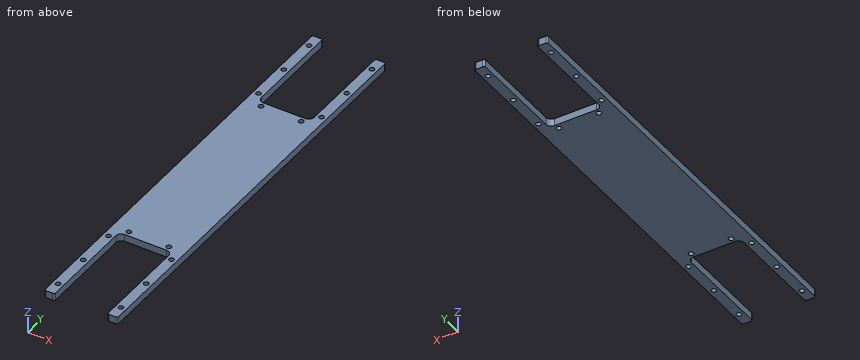
Autodesk Inventor part; units mm, degrees
ref_plane "YZ Plane" through (0, 0, 0) normal (1, 0, 0) x (0, 1, 0)
ref_plane "XZ Plane" through (0, 0, 0) normal (0, 1, 0) x (-1, 0, 0)
ref_plane "XY Plane" through (0, 0, 0) normal (0, 0, 1) x (1, 0, 0)
sketch "스케치1" plane through (0, 0, 0) normal (0, 0, 1) x (1, 0, 0)
  line L0 (-15, 14.5) -> (-11.5, 14.5)
  line L1 (-15, 14.5) -> (-20.1, 8.5)
  line L2 (-20.1, 8.5) -> (-20.1, -44.6)
  line L3 (-20.1, -44.6) -> (-15, -50.6)
  line L4 (-15, -50.6) -> (15, -50.6)
  line L5 (15, -50.6) -> (20.1, -44.6)
  line L6 (20.1, -44.6) -> (20.1, 8.5)
  line L7 (20.1, 8.5) -> (15, 14.5)
  line L8 (11.5, 14.5) -> (15, 14.5)
  arc A0 (14.5, 11.5) -> (11.5, 14.5) centre (11.5, 11.5) ccw
  line L9 (14.5, -42) -> (14.5, 11.5)
  arc A1 (11.5, -45) -> (14.5, -42) centre (11.5, -42) ccw
  line L10 (-11.5, -45) -> (11.5, -45)
  arc A2 (-14.5, -42) -> (-11.5, -45) centre (-11.5, -42) ccw
  line L11 (-14.5, 11.5) -> (-14.5, -42)
  arc A3 (-11.5, 14.5) -> (-14.5, 11.5) centre (-11.5, 11.5) ccw
  circle A4 centre (-17.3, 4) radius 1.35
  circle A5 centre (-17.3, -18) radius 1.35
  circle A6 centre (-11, -47.8) radius 1.35
  circle A7 centre (17.3, 4) radius 1.35
  circle A8 centre (17.3, -18) radius 1.35
  circle A9 centre (11, -47.8) radius 1.35
  circle A10 centre (-17.3, -40) radius 1.35
  circle A11 centre (17.3, -40) radius 1.35
  line L12 (15, -225.5) -> (11.5, -225.5)
  line L13 (15, -225.5) -> (20.1, -219.5)
  line L14 (20.1, -219.5) -> (20.1, -166.4)
  line L15 (20.1, -166.4) -> (15, -160.4)
  line L16 (15, -160.4) -> (-15, -160.4)
  line L17 (-15, -160.4) -> (-20.1, -166.4)
  line L18 (-20.1, -166.4) -> (-20.1, -219.5)
  line L19 (-20.1, -219.5) -> (-15, -225.5)
  line L20 (-11.5, -225.5) -> (-15, -225.5)
  arc A12 (-14.5, -222.5) -> (-11.5, -225.5) centre (-11.5, -222.5) ccw
  line L21 (-14.5, -169) -> (-14.5, -222.5)
  arc A13 (-11.5, -166) -> (-14.5, -169) centre (-11.5, -169) ccw
  line L22 (11.5, -166) -> (-11.5, -166)
  arc A14 (14.5, -169) -> (11.5, -166) centre (11.5, -169) ccw
  line L23 (14.5, -222.5) -> (14.5, -169)
  arc A15 (11.5, -225.5) -> (14.5, -222.5) centre (11.5, -222.5) ccw
  circle A16 centre (17.3, -215) radius 1.35
  circle A17 centre (17.3, -193) radius 1.35
  circle A18 centre (11, -163.2) radius 1.35
  circle A19 centre (-17.3, -215) radius 1.35
  circle A20 centre (-17.3, -193) radius 1.35
  circle A21 centre (-11, -163.2) radius 1.35
  circle A22 centre (17.3, -171) radius 1.35
  circle A23 centre (-17.3, -171) radius 1.35
  line L24 (20.1, -222.5) -> (20.1, 11.5)
  line L25 (-20.1, 11.5) -> (-20.1, -222.5)
  line L26 (14.5, -222.5) -> (14.5, -169)
  line L27 (11.5, -166) -> (-11.5, -166)
  line L28 (-14.5, -169) -> (-14.5, -222.5)
  arc A24 (14.5, -169) -> (11.5, -166) centre (11.5, -169) ccw
  arc A25 (-11.5, -166) -> (-14.5, -169) centre (-11.5, -169) ccw
  arc A26 (11.5, -45) -> (14.5, -42) centre (11.5, -42) ccw
  arc A27 (-14.5, -42) -> (-11.5, -45) centre (-11.5, -42) ccw
  line L29 (11.5, -45) -> (-11.5, -45)
  line L30 (-14.5, -42) -> (-14.5, 11.5)
  line L31 (14.5, 11.5) -> (14.5, -42)
  line L32 (20.1, 11.5) -> (14.5, 11.5)
  line L33 (-14.5, 11.5) -> (-20.1, 11.5)
  line L34 (-20.1, -222.5) -> (-14.5, -222.5)
  line L35 (14.5, -222.5) -> (20.1, -222.5)
  point P0 (0, 0)
  dimension "d0" = 3
extrude "판1" add sketch "스케치1" along normal blind 4 contours L33 L11 A2 L10 A1 L9 L32 L7 L6 L5 L4 L3 L2 L1 | L1 L25 L33 | L3 L4 L5 L24 L15 L16 L17 L25 | L17 L16 L15 L14 L13 L35 L23 A14 L22 A13 L21 L34 L19 L18 | L19 L34 L25 | L7 L32 L24 | L24 L35 L13
fillet "모서리 라운드1" radius 1 8 edges at (14.5, -222.5, 2) (20.1, -222.5, 2) (-14.5, -222.5, 2) (-20.1, -222.5, 2) (-20.1, 11.5, 2) (-14.5, 11.5, 2) (14.5, 11.5, 2) (20.1, 11.5, 2)
equation "\"TransitionRadius\" = BendRadius"
properties part number "bar1"
Input: part model. Units: mm. Frame: model coordinates. Coordinates: 2 decimals unless noted, no trailing zeros. Loops run counter-clockwise (first coordinate to the right, second up) from the corner with the lowest first, then second, coordinate; pieces in that order, holes last. Notation, with made-up numbers: (-15.5, 16.5) - (-0.5, 16.5) arc R13 ccw to (-0.5, 34.5) - close; hole circle Ø10 at (84.5, -28). An arc over 180 degrees is marked (long way). Answer in a Markdown table with one row per item. Add a question column.
Item 1: Contact query for flat-ended pins moving along their axis: P1, Ø2, axis at x = 17.3, y = -171, coming from the -Z side; P2, Ø3, axis at x = -11, y = -47.8, coming from the +Z side. Output: stop coordinate, or through.
Item 2: Line query: line 1 along X through (y, z) = (-215, 1.55); line 2 along X through (y, z) = (-190, 1.2); line 3 along Y through (x, z) = (-10, 2.95). Output: solid intervals per line, ascending. Write a range as [from, to].
Item 3: Section query B-B on z = 2. State how many separate pieces and enclosed holes the cut face has, then the cut area to 3 significant figures.
Item 4: Section query A-A on x = -6. Return the cut outline in (y, z).
Recorded:
| question | item | result |
|---|---|---|
| 1 | P1 | through |
| 1 | P2 | z = 4 |
| 2 | line 1 | [-20.1, -18.65], [-15.95, -14.5], [14.5, 15.95], [18.65, 20.1] |
| 2 | line 2 | [-20.1, -14.5], [14.5, 20.1] |
| 2 | line 3 | [-166, -164.11], [-162.29, -48.71], [-46.89, -45] |
| 3 | separate pieces | 1 |
| 3 | enclosed holes | 16 |
| 3 | area | 6,040 mm^2 |
| 4 | outline | (-166, 0) - (-45, 0) - (-45, 4) - (-166, 4) - close |
